from build123d import *

# Parameters (mm, degrees)
F0_W         = 63.5
F0_H         = 50.8
F1_DEPTH     = 76.2
F3_DEPTH     = 38.1
F4_T         = 2.54
F4_T3_DEPTH  = 9.906
F4_T5_DEPTH  = 46.228
F4_T7_DEPTH  = 12.7
F4_T9_DEPTH  = 12.7
F4_T11_DEPTH = 25.4
F4_T13_DEPTH = 43.18
F5_W         = 49.4960099459
F5_H         = 36.6942100227
F5_W_2       = 49.6212309226
F5_H_2       = 16.634516418
F6_DEPTH     = 1.27
F7_W         = 57.8342098743
F7_H         = 36.6147905588
F8_DEPTH     = 1.27
F10_W        = 61.5059640259
F10_H        = 33.8196810335
F11_DEPTH    = 1.27


# Not quite as in the source:
# - a shell that OpenCascade refuses in one call is made with other operations: the cavity is built on its own and cut out


with BuildPart() as f1:
    # F0 (on Top) → F1 (new body)
    with BuildSketch(Plane.XY):
        with Locations((-4.2696721688, -14.4747652373)):
            Rectangle(F0_W, F0_H)
    extrude(amount=F1_DEPTH)

    # F2 (on face) → F3 (cut)
    with BuildSketch(Plane.XZ.offset(39.8747652373)):
        Polygon((9.9543278312, 58.42), (-31.1936721688, 58.42), (-31.1936721688, 50.8), (-39.8653410375, 50.8), (-39.8653410375, 45.72), (-31.1936721688, 45.72), (-31.1936721688, 38.1), (9.9543278312, 38.1), align=None)
    extrude(amount=-F3_DEPTH, mode=Mode.SUBTRACT)

    # F4: shell of thickness 2.54, made by hand


with BuildPart() as f4_core1:
    # F4_t2: copy of F1
    add(f1.part)

    # the walls: a layer under each face that stays
    f4_faces = [f4_core1.faces().sort_by_distance(p)[0] for p in [
        (-4.2696721688, 10.9252347627, 38.1),
        (27.4803278312, -14.4747652373, 38.1),
        (-36.0196721688, -14.4747652373, 38.1),
        (-4.2696721688, -14.4747652373, 0),
        (-4.2696721688, -14.4747652373, 76.2),
        (-33.6066721688, -20.8247652373, 45.72),
        (-13.0326721688, -1.7747652373, 48.26),
        (-33.6066721688, -20.8247652373, 50.8),
        (-31.1936721688, -20.8247652373, 54.61),
        (-10.6196721688, -20.8247652373, 58.42),
        (9.9543278312, -20.8247652373, 48.26),
        (-10.6196721688, -20.8247652373, 38.1),
        (-31.1936721688, -20.8247652373, 41.91),
    ]]
    thicken(f4_faces, amount=-F4_T, mode=Mode.SUBTRACT)

    # F4_s4 → F4_t3 (cut)
    with BuildSketch(Plane.YZ.offset(-38.5596721688)):
        Polygon((-1.8001652373, 45.7454), (-1.7747652373, 43.18), (0.7652347627, 43.18), (0.7652347627, 45.72), align=None)
        Polygon((-1.8001652373, 50.7746), (0.7652347627, 50.8), (0.7652347627, 53.34), (-1.7747652373, 53.34), align=None)
    extrude(amount=F4_T3_DEPTH, mode=Mode.SUBTRACT)

    # F4_s6 → F4_t5 (cut)
    with BuildSketch(Plane.YZ.offset(-33.7336721688)):
        Polygon((-1.8001652373, 38.1254), (0.7652347627, 38.1), (0.7652347627, 35.56), (-1.7747652373, 35.56), align=None)
        Polygon((-1.8001652373, 58.3946), (0.7652347627, 58.42), (0.7652347627, 60.96), (-1.7747652373, 60.96), align=None)
    extrude(amount=F4_T5_DEPTH, mode=Mode.SUBTRACT)

    # F4_s8 → F4_t7 (cut)
    with BuildSketch(Plane.XY.offset(35.56)):
        Polygon((-31.1682721688, -1.8001652373), (-31.1936721688, 0.7652347627), (-33.7336721688, 0.7652347627), (-33.7336721688, -1.7747652373), align=None)
    extrude(amount=F4_T7_DEPTH, mode=Mode.SUBTRACT)

    # F4_s10 → F4_t9 (cut)
    with BuildSketch(Plane.XY.offset(48.26)):
        Polygon((-31.1682721688, -1.8001652373), (-31.1936721688, 0.7652347627), (-33.7336721688, 0.7652347627), (-33.7336721688, -1.7747652373), align=None)
    extrude(amount=F4_T9_DEPTH, mode=Mode.SUBTRACT)

    # F4_s12 → F4_t11 (cut)
    with BuildSketch(Plane.XY.offset(35.56)):
        Polygon((9.9289278312, -1.8001652373), (9.9543278312, 0.7652347627), (12.4943278312, 0.7652347627), (12.4943278312, -1.7747652373), align=None)
    extrude(amount=F4_T11_DEPTH, mode=Mode.SUBTRACT)

    # F4_s14 → F4_t13 (cut)
    with BuildSketch(Plane.XZ.offset(-0.7652347627)):
        Polygon((-31.1682721688, 58.3946), (-33.7336721688, 58.42), (-33.7336721688, 60.96), (-31.1936721688, 60.96), align=None)
        Polygon((9.9289278312, 58.3946), (9.9543278312, 60.96), (12.4943278312, 60.96), (12.4943278312, 58.42), align=None)
        Polygon((9.9289278312, 38.1254), (12.4943278312, 38.1), (12.4943278312, 35.56), (9.9543278312, 35.56), align=None)
        Polygon((-31.1682721688, 38.1254), (-31.1936721688, 35.56), (-33.7336721688, 35.56), (-33.7336721688, 38.1), align=None)
    extrude(amount=F4_T13_DEPTH, mode=Mode.SUBTRACT)


with BuildPart() as f1_1:
    add(f1.part)

    # what is left inside the walls is the cavity
    f4_cavity = [f4_core1.part.solids().sort_by_distance(p)[0] for p in [
        (-4.269672, 8.359835, 49.953333),
    ]]
    add(f4_cavity, mode=Mode.SUBTRACT)

    # F5 (on Right) → F6 (join, symmetric)
    with BuildSketch(Plane.YZ):
        with Locations((-15.0325410068, 18.3471050113)):
            Rectangle(F5_W, F5_H)
        with Locations((-15.3072369285, 67.7350275218)):
            Rectangle(F5_W_2, F5_H_2)
    extrude(amount=F6_DEPTH, both=True)

    # F7 (on Front) → F8 (join, symmetric)
    with BuildSketch(Plane.XZ):
        with Locations((-4.0594032034, 18.3073952794)):
            Rectangle(F7_W, F7_H)
    extrude(amount=F8_DEPTH, both=True)

    # F10 (on offset) → F11 (join, symmetric)
    with BuildSketch(Plane.XZ.offset(27.94)):
        with Locations((-4.893549718, 19.6837866679)):
            Rectangle(F10_W, F10_H)
    extrude(amount=F11_DEPTH, both=True)


solid = f1_1.part
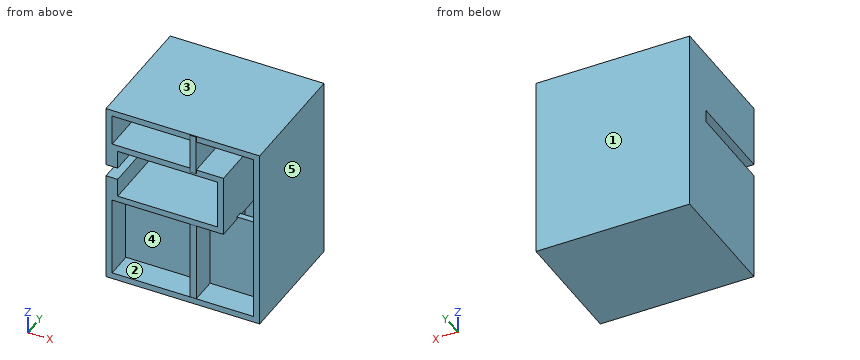
Could you check a few things on this model? Use its own coordinates, in mm. Face numbers are marked on the shaded views. A direction names the side the tool comes from. Coordinates: 2 decimals unless noted, no trailing zeros. Order: outer loops, then holes, each group sorted by start corner. A loop starts at its lowest first (then second) coordinate and runs counter-clockwise, first axis right, second up.
Q1. Which directions (+Z, -Z, +X, -X, +Y, -Y) give clear straight access to the entire face, cutting with the end or side of a thin tool? Please do the marked faces 4 and 5.
Q2. Will these pins go through, and if not, where does the flat tip stop? pin 1 (12 mm diameter, centred on x = 10.5, z = 11.5, fed in from -Y); pin 2 (1 mm diameter, centred on x = -11.5, z = 42, fed in from -Y); pin 3 (10 mm diameter, centred on x = 0, z = 55, fed in from -Y).
Q3. Thinking about a two-plate mould opening in Y: for the marked faces 1, 2 and 3, which applies, released by +Y, released by -Y, zero draft, split by the parting line, or undercut?
Q4. Suppose I cut it at A-A on x = 14.5. Please give me the cut outline in (y, z).
Q5. Suppose I cut it at C-C on z = 29.5. Please give me the cut outline in (x, y).
Q6. Please list where these lines run through material, in increasing order: L1, parallel to X at y = -22, z = 52.5; L2, parallel to X at y = -8, z = 63.5; L3, parallel to Y at x = -22.5, z = 22.
Q7. Suppose I cut it at D-D on z = 41.5. Please give me the cut outline in (x, y).
Q8. Suppose I cut it at B-B on y = -28. Give the number of separate pieces and of enclosed holes in the cut face, and give its area (3 significant figures).
Answer:
1. face 4: -Y
1. face 5: +Z, -Z, +X, +Y, -Y
2. pin 1: stops at y = -29.21
2. pin 2: stops at y = -1.77
2. pin 3: stops at y = -40.12
3. face 1: released by +Y
3. face 2: undercut
3. face 3: zero draft
4. outline: (-39.87, 0) - (10.93, 0) - (10.93, 76.2) - (-39.87, 76.2) - (-39.87, 73.66) - (8.39, 73.66) - (8.39, 2.54) - (1.27, 2.54) - (1.27, 36.61) - (-1.27, 36.61) - (-1.27, 2.54) - (-39.87, 2.54) - close; (-29.21, 2.77) - (-26.67, 2.77) - (-26.67, 36.59) - (-29.21, 36.59) - close
5. outline: (-36.02, -39.87) - (-33.48, -39.87) - (-33.48, -29.21) - (-1.27, -29.21) - (-1.27, -39.78) - (1.27, -39.78) - (1.27, -29.21) - (24.94, -29.21) - (24.94, -39.87) - (27.48, -39.87) - (27.48, 10.93) - (-36.02, 10.93) - close; hole (-33.48, -26.67) - (-1.27, -26.67) - (-1.27, -1.27) - (-32.98, -1.27) - (-32.98, 1.27) - (-1.27, 1.27) - (-1.27, 8.39) - (-33.48, 8.39) - close; hole (1.27, -26.67) - (24.94, -26.67) - (24.94, 8.39) - (1.27, 8.39) - (1.27, 1.27) - (24.86, 1.27) - (24.86, -1.27) - (1.27, -1.27) - close
6. L1: x = -36.02 to -31.19, 9.95 to 12.49, 24.94 to 27.48
6. L2: x = -36.02 to -33.48, -1.27 to 1.27, 24.94 to 27.48
6. L3: y = -29.21 to -26.67, -1.27 to 1.27, 8.39 to 10.93
7. outline: (-36.02, -39.87) - (-31.19, -39.87) - (-31.19, -1.77) - (9.95, -1.77) - (9.95, -39.87) - (12.49, -39.87) - (12.49, 0.77) - (-33.48, 0.77) - (-33.48, 8.39) - (24.94, 8.39) - (24.94, -39.87) - (27.48, -39.87) - (27.48, 10.93) - (-36.02, 10.93) - close
8. separate pieces: 1
8. enclosed holes: 4
8. area: 2,950 mm2
